from build123d import *

# Parameters (mm, degrees)
SKETCH2_R           = 19.05
BOSS_EXTRUDE1_DEPTH = 50.8
SKETCH3_R           = 2.593311049
SKETCH3_R_2         = 2.552831608
SKETCH3_R_3         = 2.477244579
SKETCH3_R_4         = 2.54595384
CUT_EXTRUDE1_DEPTH  = 67.295946332


with BuildPart() as part:
    # Sketch2 → Boss-Extrude1 (new body)
    with BuildSketch(Plane.XY):
        Circle(SKETCH2_R)
    extrude(amount=BOSS_EXTRUDE1_DEPTH)

    # Sketch3 → Cut-Extrude1 (cut, through all)
    with BuildSketch(Plane.ZY.offset(19.05)):
        with Locations((5.08, 0)):
            Circle(SKETCH3_R)
        with Locations((12.7, 0)):
            Circle(SKETCH3_R_2)
        with Locations((45.663499475, 0)):
            Circle(SKETCH3_R_3)
        with Locations((38.043499475, 0)):
            Circle(SKETCH3_R_4)
    extrude(amount=-CUT_EXTRUDE1_DEPTH, mode=Mode.SUBTRACT)


solid = part.part
Verification items for the finished model (mm, model axes). Round coordinates to 2 decimals unless told otherwise and drop trailing zeros. Loops run counter-clockwise (first coordinate to the right, second up) from the corner with the lowest first, then second, coordinate; pieces in that order, holes last. Notation, with made-up numbers: (82.25, 20.25) - (101.25, 20.25) arc R25 ccw to (101.25, 34.25) - close; hole circle Ø5 at (8, -36). An arc over 180 degrees is marked (long way). Answer in a Markdown table with one row per item. Add a question column.
Q1. Section check B-B on y = 0. Enter the section's corners in (x, z).
Q2. Section check C-C on z = 12.7. Enter the section's corners in (x, y), plus the area to 3 significant figures.
Q3. Section check D-D on x = 14.5. Enter the section's corners in (y, z), plus the area to 3 significant figures.
Q4. Section check A-A on x = 0. Enter the section's corners in (y, z).
Q5. Release check for a two-part mould opening along Z. For faces 1 (the face through (0, 0, 0)), 2 (the face through (-0.267, -0.975, 40.395)), 3 (the face through (0, 0, 50.8)) record: pulls with the +Z half, pulls with the -Z half, needs draft (parallel to the pull), parting line crosses it, or undercut.
Q6. Gauge pin test, flat ends, axial feed: pin 1 (4 mm diameter, centred on x = -3.5, z = 35, fed in from +Y); pin 2 (2 mm diameter, centred on x = 3.5, z = 8, fed in from -Y); pin 3 (3 mm diameter, centred on y = -10, z = 16, fed in from +X). Record the tip position at first contact, or that the pin passes through.
Q7. Material ranges on line 1 (Z direction, x = 7, y = 0); line 2 (Z direction, x = -11, y = -1.5); line 3 (Y direction, x = 2, z = 5), recorded low to high.
Found:
| question | item | result |
|---|---|---|
| 1 | outline | (-19.05, 0) - (19.05, 0) - (19.05, 2.49) - (-19.05, 2.49) - close; (-19.05, 7.67) - (19.05, 7.67) - (19.05, 10.15) - (-19.05, 10.15) - close; (-19.05, 15.25) - (19.05, 15.25) - (19.05, 35.5) - (-19.05, 35.5) - close; (-19.05, 40.59) - (19.05, 40.59) - (19.05, 43.19) - (-19.05, 43.19) - close; (-19.05, 48.14) - (19.05, 48.14) - (19.05, 50.8) - (-19.05, 50.8) - close |
| 2 | outline | (-18.88, -2.55) arc R19.05 ccw to (18.88, -2.55) - close; (-18.88, 2.55) - (18.88, 2.55) arc R19.05 ccw to start |
| 2 | area | 946 mm² |
| 3 | outline | (-12.36, 0) - (12.36, 0) - (12.36, 50.8) - (-12.36, 50.8) - close; hole circle Ø5.19 at (0, 5.08); hole circle Ø5.11 at (0, 12.7); hole circle Ø5.09 at (0, 38.04); hole circle Ø4.95 at (0, 45.66) |
| 3 | area | 1,170 mm² |
| 4 | outline | (-19.05, 0) - (19.05, 0) - (19.05, 50.8) - (-19.05, 50.8) - close; hole circle Ø5.19 at (0, 5.08); hole circle Ø5.11 at (0, 12.7); hole circle Ø5.09 at (0, 38.04); hole circle Ø4.95 at (0, 45.66) |
| 5 | face 1 | pulls with the -Z half |
| 5 | face 2 | undercut |
| 5 | face 3 | pulls with the +Z half |
| 6 | pin 1 | stops at y = 18.99 |
| 6 | pin 2 | stops at y = -18.89 |
| 6 | pin 3 | stops at x = 17.05 |
| 7 | line 1 | z = 0 to 2.49, 7.67 to 10.15, 15.25 to 35.5, 40.59 to 43.19, 48.14 to 50.8 |
| 7 | line 2 | z = 0 to 2.96, 7.2 to 10.63, 14.77 to 35.99, 40.1 to 43.69, 47.63 to 50.8 |
| 7 | line 3 | y = -18.94 to -2.59, 2.59 to 18.94 |
